```python
from build123d import *

# Parameters (mm, degrees)
BOSS_EXTRUDE1_DEPTH = 1.95


with BuildPart() as part:
    # Sketch1 → Boss-Extrude1 (new body)
    with BuildSketch(Plane(origin=(0, 0, 0), x_dir=(1, 0, 0), z_dir=(0, 1, 0))):
        with BuildLine():
            Line((0, -26.575), (130.828205579, -26.575))
            ThreePointArc((130.828205579, -26.575), (132.830371988, -13.354485299), (133.5, 0))
            ThreePointArc((133.5, 0), (132.830371988, 13.354485299), (130.828205579, 26.575))
            Line((130.828205579, 26.575), (0, 26.575))
            ThreePointArc((0, 26.575), (-26.575, 0), (0, -26.575))
        make_face()
    extrude(amount=BOSS_EXTRUDE1_DEPTH)


solid = part.part
```
Here's how the part is built. I have some questions about the finished solid (model axes, mm). Round coordinates to 2 decimals unless told otherwise and drop trailing zeros. Order: outer loops, then holes, each group sorted by start corner. A loop starts at its lowest first (then second) coordinate and runs counter-clockwise, first axis right, second up. Notation, with made-up numbers: (-11, -28.75) -> (26, -28.75) arc R6 ccw to (26, -18.75) -> close; hole circle Ø5 at (78.5, 41.25). An arc over 180 degrees is marked (long way). Use a Markdown table: item, result. Add a question column.
(1) Suppose I cut it at B-B, the plane z = 16. Please give me the cut outline in (x, y), and give its area (3 significant figures).
(2) Suppose I cut it at A-A, the plane y = 1.35. Please give me the cut outline in (x, z) (3 decimals), and give its area (3 significant figures).
(3) Suppose I cut it at C-C, the plane x = -11. Please give me the cut outline in (y, z), and give its area (3 significant figures).
(4) I need wall thicknesses on line 1 along X through (y, z) = (0.6, 1); line 2 along X through (y, z) = (1.2, -23); line 3 along Z through (x, y) = (-6, 0.5). Which ranges of each line are inside material? Lowest first, please.
Verdict:
| question | item | result |
|---|---|---|
| 1 | outline | (-21.22, 0) -> (132.54, 0) -> (132.54, 1.95) -> (-21.22, 1.95) -> close |
| 1 | area | 300 mm2 |
| 2 | outline | (0, -26.575) -> (130.828, -26.575) arc R133.5 ccw to (130.828, 26.575) -> (0, 26.575) arc R26.575 ccw to start |
| 2 | area | 8,160 mm2 |
| 3 | outline | (0, -24.19) -> (1.95, -24.19) -> (1.95, 24.19) -> (0, 24.19) -> close |
| 3 | area | 94.3 mm2 |
| 4 | line 1 | -26.56 to 133.5 |
| 4 | line 2 | -13.31 to 131.5 |
| 4 | line 3 | -25.89 to 25.89 |
